Here's how the part is built. I have some questions about the finished solid (model axes, mm). Face numbers are marked on the shaded views. A direction names the side the tool comes from. Round coordinates to 2 decimals unless told otherwise and drop trailing zeros. Write each loop counter-clockwise with the first axis right and the second up, starting at its lowest first coordinate (ties: lowest second). Pieces come first, ordered by that corner, then holes. Notation, with made-up numbers: (-33.5, 3) -> (12.5, 3) arc R22 ccw to (12.5, 31) -> close; hole circle Ø11 at (-23.5, 58). An arc over 180 degrees is marked (long way). Answer in a Markdown table with one row per item.
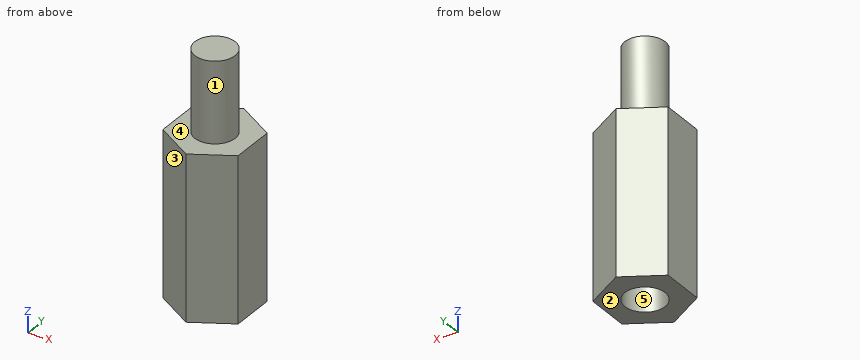
from build123d import *

# Parameters (mm, degrees)
F1_DEPTH = 12.2
F2_D     = 3
F2_DEPTH = 7.5
F2_TIP   = 0.9012909285
F3_R     = 1.5
F4_DEPTH = 6


with BuildPart() as f1:
    # F0 (on Top) → F1 (new body)
    with BuildSketch(Plane.XY):
        Polygon((2.8, -1.6165807537), (2.8, 1.6165807537), (0, 3.2331615075), (-2.8, 1.6165807537), (-2.8, -1.6165807537), (0, -3.2331615075), align=None)
    extrude(amount=F1_DEPTH)

    # F2
    with Locations(Plane(origin=(0, 0, 0), x_dir=(1, 0, 0), z_dir=(0, 0, -1))):
        with Locations((0, 0)):
            Hole(F2_D / 2, depth=F2_DEPTH)
            with Locations((0, 0, -(F2_DEPTH + F2_TIP / 2))):  # 118° drill point
                Cone(0, F2_D / 2, F2_TIP, mode=Mode.SUBTRACT)

    # F3 (on face) → F4 (join)
    with BuildSketch(Plane.XY.offset(12.2)):
        Circle(F3_R)
    extrude(amount=F4_DEPTH)


solid = f1.part
1) I want a section at B-B, the plane z = 17. List the corners of the cut face in (x, y) for me, and give its area (3 significant figures).
Response:
| item | result |
|---|---|
| outline | circle Ø3 at (0, 0) |
| area | 7.07 mm^2 |
2) I want a section at A-A, the plane z = 1.5. List the corners of the cut face in (x, y) for me, and give its area (3 significant figures).
Response:
| item | result |
|---|---|
| outline | (-2.8, -1.62) -> (0, -3.23) -> (2.8, -1.62) -> (2.8, 1.62) -> (0, 3.23) -> (-2.8, 1.62) -> close; hole circle Ø3 at (0, 0) |
| area | 20.1 mm^2 |
3) For pin 1 (3 mm diameter, centred on x = 1, y = -1, fed in from -Z); pin 2 (2 mm diameter, centred on y = 0, z = 15.5, fed in from +X), each with a flat end and sliding along its axis, tell me the tip position at first contact or that it passes through.
Response:
| item | result |
|---|---|
| pin 1 | stops at z = 0 |
| pin 2 | stops at x = 1.5 |
4) I want a section at C-C, the plane y = -2. List the corners of the cut face in (x, z) for me, and give its area (3 significant figures).
Response:
| item | result |
|---|---|
| outline | (-2.14, 0) -> (2.14, 0) -> (2.14, 12.2) -> (-2.14, 12.2) -> close |
| area | 52.1 mm^2 |
5) I need wall thicknesses on line 1 (Z direction, x = -1.25, y = -1.25); line 2 (Y direction, x = -0.2, z = 3); line 3 (Y direction, x = 1.25, z = 14). Which ranges of each line are inside material? Lowest first, please. Write a range as [from, to].
Response:
| item | result |
|---|---|
| line 1 | z = [0, 12.2] |
| line 2 | y = [-3.12, -1.49], [1.49, 3.12] |
| line 3 | y = [-0.83, 0.83] |
6) Which directions (+Z, -Z, +X, -X, +Y, -Y) give clear straight access to the entire face, cutting with the end or side of a thin tool? Please do the marked faces 1 and 2.
Response:
| item | result |
|---|---|
| face 1 | +Z |
| face 2 | -Z, +X, -X, +Y, -Y |
7) We'd pull the mould along X, two halves only. Please class the marked faces 3, 4 and 5: +X half, -X half, draft (parallel to the pull), parting line (faces both ways), or undercut.
Response:
| item | result |
|---|---|
| face 3 | -X half |
| face 4 | draft |
| face 5 | undercut |
